Input: part model. Units: mm. Frame: model coordinates. Face numbers are marked on the shaded views. A direction names the side the tool comes from. Coordinates: 2 decimals unless noted, no trailing zeros. Write each loop counter-clockwise with the first axis right and the second up, starting at its lowest first coordinate (ties: lowest second). Pieces come first, ordered by that corner, then holes. Notation, with made-up numbers: M 6,8 L 52,8 A11 cw 52,13 Z; hole C -33,-2.75 d10. An arc over 180 degrees is marked long. Write each question's results on one line, items separated by ' | '. Start each with the question number.
1. Set-up query: the marked faces 1, 2 and 3. Return all of +Z, -Z, +X, -X, +Y, -Y with unobstructed straight access to the full face (end or side cutting, diameter ignored); none if empty.
2. Section query B-B, the plane z = 17.5. Output: boundary loops of the cut face in (x, y), and give its area (3 significant figures).
3. Section query D-D, the plane x = -10. Output: boundary loops of the cut face in (y, z).
4. Ray query, probe 1 along Y at (x, z) = (0, 17.5); probe 2 along X at (y, z) = (0.5, 18); probe 3 along X at (y, z) = (3.5, 10.5). Return the intervals inside material, ascending.
5. First-contact query: pin 1 (8 mm diameter, centred on x = -0.5, y = -7.5, fed in from +Z); pin 2 (9 mm diameter, centred on x = 16.5, z = 15.5, fed in from -Y); pin 3 (6 mm diameter, centred on x = -10.5, z = 8, fed in from -Y). Flat tips, straight axial feed; report the tip coordinate or a pass-through.
6. Section query C-C, the plane x = 0. Output: boundary loops of the cut face in (y, z).
7. Pull-direction query (X, two-part tool) for the marked faces 4, 5 and 6; classes: +X half, -X half, draft (parallel to the pull), parting line (faces both ways), or undercut.
8. Section query A-A, the plane y = 0. Output: boundary loops of the cut face in (x, z), and give its area (3 significant figures).
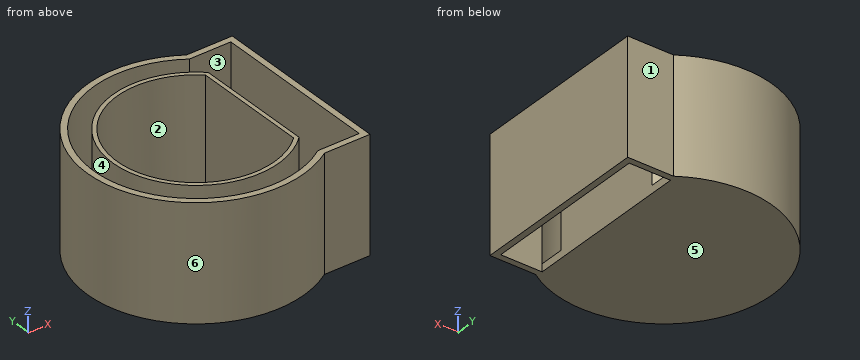
```python
from build123d import *

# Parameters (mm, degrees)
F1_DEPTH = 1.5
F2_DEPTH = 22.5
F4_DEPTH = 25


# Not quite as in the source:
# - a feature names something its author has since deleted; it is built from what else it names


with BuildPart() as f1:
    # F0 (on Top) → F1 (new body)
    with BuildSketch(Plane.XY):
        with BuildLine():
            Line((20.6026545555, 17.7), (11.6683332143, 17.7))
            ThreePointArc((11.6683332143, 17.7), (-21.2, 0), (11.6683332143, -17.7))
            Line((11.6683332143, -17.7), (20.6026545555, -17.7))
            Line((20.6026545555, -17.7), (20.6026545555, 17.7))
        make_face()
        with BuildLine():
            ThreePointArc((11.3026545555, -16.5), (-20, 0), (11.3026545555, 16.5))
            Line((11.3026545555, 16.5), (19.4026545555, 16.5))
            Line((19.4026545555, 16.5), (19.4026545555, -16.5))
            Line((19.4026545555, -16.5), (11.3026545555, -16.5))
        make_face(mode=Mode.SUBTRACT)
        with BuildLine():
            Line((19.4026545555, 16.5), (11.3026545555, 16.5))
            ThreePointArc((11.3026545555, 16.5), (-20, 0), (11.3026545555, -16.5))
            Line((11.3026545555, -16.5), (19.4026545555, -16.5))
            Line((19.4026545555, -16.5), (19.4026545555, 16.5))
        make_face()
        with BuildLine():
            ThreePointArc((11.3026545555, -11.6752944288), (-16.25, 0), (11.3026545555, 11.6752944288))
            Line((11.3026545555, 11.6752944288), (11.3026545555, -11.6752944288))
        make_face(mode=Mode.SUBTRACT)
        with BuildLine():
            Line((11.3026545555, -11.6752944288), (11.3026545555, 11.6752944288))
            ThreePointArc((11.3026545555, 11.6752944288), (-16.25, 0), (11.3026545555, -11.6752944288))
        make_face()
        with BuildLine():
            ThreePointArc((10.5026545555, -11.3312288517), (-15.45, 0), (10.5026545555, 11.3312288517))
            Line((10.5026545555, 11.3312288517), (10.5026545555, -11.3312288517))
        make_face(mode=Mode.SUBTRACT)
        with BuildLine():
            Line((10.5026545555, -11.3312288517), (10.5026545555, 11.3312288517))
            ThreePointArc((10.5026545555, 11.3312288517), (-15.45, 0), (10.5026545555, -11.3312288517))
        make_face()
    extrude(amount=F1_DEPTH)

    # F0 (on Top) → F2 (join)
    with BuildSketch(Plane.XY):
        with BuildLine():
            Line((20.6026545555, 17.7), (11.6683332143, 17.7))
            ThreePointArc((11.6683332143, 17.7), (-21.2, 0), (11.6683332143, -17.7))
            Line((11.6683332143, -17.7), (20.6026545555, -17.7))
            Line((20.6026545555, -17.7), (20.6026545555, 17.7))
        make_face()
        with BuildLine():
            ThreePointArc((11.3026545555, -16.5), (-20, 0), (11.3026545555, 16.5))
            Line((11.3026545555, 16.5), (19.4026545555, 16.5))
            Line((19.4026545555, 16.5), (19.4026545555, -16.5))
            Line((19.4026545555, -16.5), (11.3026545555, -16.5))
        make_face(mode=Mode.SUBTRACT)
        with BuildLine():
            Line((11.3026545555, -11.6752944288), (11.3026545555, 11.6752944288))
            ThreePointArc((11.3026545555, 11.6752944288), (-16.25, 0), (11.3026545555, -11.6752944288))
        make_face()
        with BuildLine():
            ThreePointArc((10.5026545555, -11.3312288517), (-15.45, 0), (10.5026545555, 11.3312288517))
            Line((10.5026545555, 11.3312288517), (10.5026545555, -11.3312288517))
        make_face(mode=Mode.SUBTRACT)
    extrude(amount=F2_DEPTH)

    # F3 (on face) → F4 (cut)
    with BuildSketch(Plane.XY.offset(1.5)):
        Polygon((19.4026545555, 16.5), (11.3026545555, 16.5), (11.3026545555, 11.6752944288), (11.3026545555, -11.6752944288), (11.3026545555, -16.5), (19.4026545555, -16.5), align=None)
    extrude(amount=-F4_DEPTH, mode=Mode.SUBTRACT)


solid = f1.part
```
Answer:
1) face 1: +Z, -Z, +X, +Y | face 2: +Z | face 3: +Z, -Z
2) outline: M 11.3,-11.68 L 11.3,11.68 A16.25 ccw long Z; M 11.67,-17.7 L 20.6,-17.7 L 20.6,17.7 L 11.67,17.7 A21.2 ccw long Z; hole M 10.5,-11.33 L 10.5,11.33 A15.45 ccw long Z; hole M 11.3,-16.5 L 19.4,-16.5 L 19.4,16.5 L 11.3,16.5 A20 ccw long Z | area: 246 mm^2
3) outline: M -18.69,0 L 18.69,0 L 18.69,22.5 L 17.32,22.5 L 17.32,1.5 L 12.81,1.5 L 12.81,22.5 L 11.78,22.5 L 11.78,1.5 L -11.78,1.5 L -11.78,22.5 L -12.81,22.5 L -12.81,1.5 L -17.32,1.5 L -17.32,22.5 L -18.69,22.5 Z
4) probe 1: -21.2 to -20, -16.25 to -15.45, 15.45 to 16.25, 20 to 21.2 | probe 2: -21.19 to -19.99, -16.24 to -15.44, 10.5 to 11.3, 19.4 to 20.6 | probe 3: -20.91 to -19.69, -15.87 to -15.05, 10.5 to 11.3, 19.4 to 20.6
5) pin 1: z = 1.5 | pin 2: y = -17.7 | pin 3: y = -19.83
6) outline: M -21.2,0 L 21.2,0 L 21.2,22.5 L 20,22.5 L 20,1.5 L 16.25,1.5 L 16.25,22.5 L 15.45,22.5 L 15.45,1.5 L -15.45,1.5 L -15.45,22.5 L -16.25,22.5 L -16.25,1.5 L -20,1.5 L -20,22.5 L -21.2,22.5 Z
7) face 4: undercut | face 5: draft | face 6: parting line
8) outline: M -21.2,0 L 11.3,0 L 11.3,22.5 L 10.5,22.5 L 10.5,1.5 L -15.45,1.5 L -15.45,22.5 L -16.25,22.5 L -16.25,1.5 L -20,1.5 L -20,22.5 L -21.2,22.5 Z; M 19.4,0 L 20.6,0 L 20.6,22.5 L 19.4,22.5 Z | area: 135 mm^2
